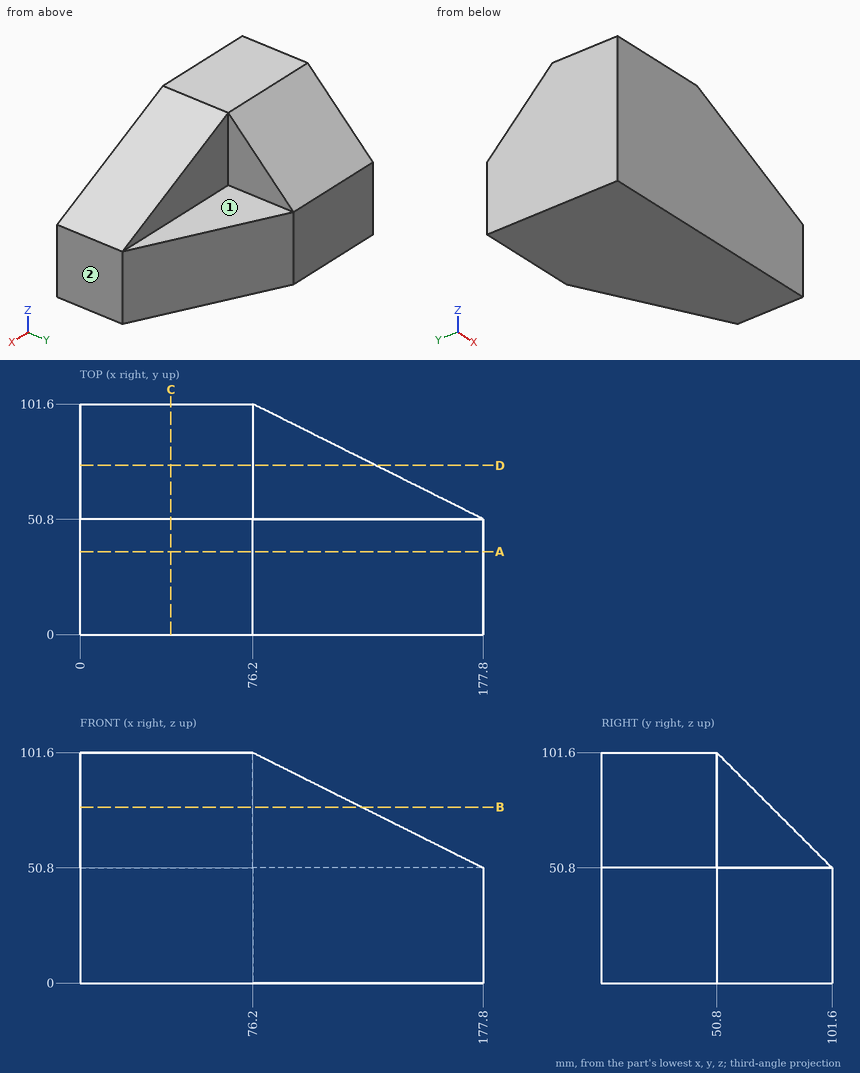
Here's the drawing with two shaded views (mm, measured from the low corner). I have some questions. A direction names the side the tool comes from. Round coordinates to 2 decimals unless told otherwise and drop trailing zeros. Write each loop counter-clockwise with the first axis right and the second up, starting at its lowest first coordinate (ties: lowest second). Pieces come first, ordered by that corner, then holes.
(1) Which directions (+Z, -Z, +X, -X, +Y, -Y) give clear straight access to the entire face, cutting with the end or side of a thin tool? Please do the marked faces 1 and 2.
Findings below:
face 1: +Z, +X, +Y
face 2: +Z, -Z, +X, +Y, -Y
(2) Suppose I cut it at D-D on y = 74.5. Write out the boundary of the cut face in (x, z).
Findings below:
outline: (0, 0) - (130.4, 0) - (130.4, 50.8) - (76.2, 50.8) - (76.2, 77.9) - (0, 77.9) - close
(3) For pin 1 (4 mm diameter, centred on y = 46.5, z = 26.5, fed in from -X); pin 2 (15 mm diameter, centred on y = 64.5, z = 71.5, fed in from +X); pin 3 (2 mm diameter, centred on x = 94.5, y = 35.5, fed in from +Z); pin 4 (6 mm diameter, centred on y = 78.5, z = 45.5, fed in from +X), each with a flat end and sliding along its axis, tell me the tip position at first contact or that it passes through.
Findings below:
pin 1: stops at x = 0
pin 2: stops at x = 76.2
pin 3: stops at z = 92.95
pin 4: stops at x = 128.4
(4) Suppose I cut it at A-A on y = 36.5. Write out the boundary of the cut face in (x, z).
Findings below:
outline: (0, 0) - (177.8, 0) - (177.8, 50.8) - (76.2, 101.6) - (0, 101.6) - close
(5) If I drill on probe 1 along Y at (x, z) = (102, 76); probe 2 along X at (y, z) = (92, 54); probe 3 along Y at (x, z) = (10, 93), over which ranges is the centre line in solid material (lowest first)?
Findings below:
probe 1: y = 0 to 50.8
probe 2: x = 0 to 76.2
probe 3: y = 0 to 59.4
(6) Suppose I cut it at C-C on x = 40. Write out the boundary of the cut face in (y, z).
Findings below:
outline: (0, 0) - (101.6, 0) - (101.6, 50.8) - (50.8, 101.6) - (0, 101.6) - close
(7) Suppose I cut it at B-B on z = 77.5. Write out the boundary of the cut face in (x, y).
Findings below:
outline: (0, 0) - (124.4, 0) - (124.4, 50.8) - (76.2, 50.8) - (76.2, 74.9) - (0, 74.9) - close
